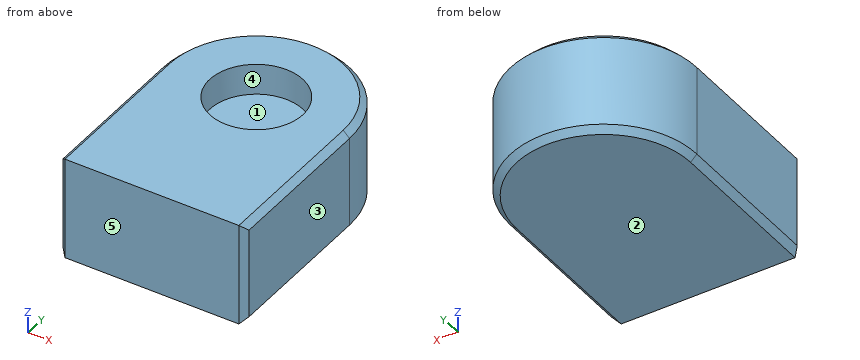
from build123d import *

# Parameters (mm, degrees)
EXTRUDE_1_DEPTH     = 16.5
CHAMFER_1_SIZE      = 1
SKETCH_2_R          = 7.5
CUT_EXTRUDE_1_DEPTH = 5


with BuildPart() as part:
    # 草圖1 → 填料-伸長1 (new body)
    with BuildSketch(Plane.XY):
        with BuildLine():
            Line((-15, 0), (-15, -26))
            Line((-15, -26), (15, -26))
            Line((15, -26), (15, 0))
            ThreePointArc((15, 0), (0, 15), (-15, 0))
        make_face()
    extrude(amount=EXTRUDE_1_DEPTH)

    # 導角1
    chamfer_1_edges = [part.edges().sort_by_distance(p)[0] for p in [
        (15, -13, 16.5),
        (0, 15, 16.5),
        (15, -13, 0),
        (-15, -13, 0),
        (0, 15, 0),
        (-15, -13, 16.5),
        (15, -26, 8.25),
        (-15, -26, 8.25),
    ]]
    chamfer(chamfer_1_edges, length=CHAMFER_1_SIZE)

    # 草圖2 → 除料-伸長1 (cut)
    with BuildSketch(Plane.XY.offset(16.5)):
        Circle(SKETCH_2_R)
    extrude(amount=-CUT_EXTRUDE_1_DEPTH, mode=Mode.SUBTRACT)


solid = part.part
Check sheet for the modelled part. Datum: model origin and axes. Units: mm. Face numbers are marked on the shaded views. A direction names the side the tool comes from. Round coordinates to 2 decimals unless told otherwise and drop trailing zeros. Loops run counter-clockwise (first coordinate to the right, second up) from the corner with the lowest first, then second, coordinate; pieces in that order, holes last.
1. Scan lines: probe 1 along Y at (x, z) = (0, 13.1); probe 2 along Z at (x, y) = (3, 6); probe 3 along X at (y, z) = (0.5, 15.5). Record each from-to range of solid material in increasing order.
2. Sectioned sample at A-A on z = 3. Record the boundary of the cut face in (x, y).
3. Set-up check for the marked faces 1 and 2: record each of +Z, -Z, +X, -X, +Y, -Y from which the full face is reachable in a straight line by a thin tool's end or side.
4. Mould release check, pull along Y, two halves, no side actions. Record for the marked faces 3, 4 and 5: released by +Y, released by -Y, zero draft, split by the parting line, or undercut.
5. Sectioned sample at B-B on x = 0. Record the boundary of the cut face in (y, z).
6. Gauge pin test, flat ends, axial feed: pin 1 Ø3 at (x, z) = (11, 10.5) entering from +Y; pin 2 Ø16.5 at (x, y) = (-2.5, 1) entering from +Z; pin 3 Ø2 at (x, z) = (7, 7) entering from +Y; pin 4 Ø2 at (y, z) = (5, 13) entering from +X. Record the tip position at first contact, or that the pin passes through.
Recorded:
1. probe 1: y = -26 to -7.5, 7.5 to 15
1. probe 2: z = 0 to 11.5
1. probe 3: x = -14.99 to -7.48, 7.48 to 14.99
2. outline: (-15, -25) - (-14, -26) - (14, -26) - (15, -25) - (15, 0) arc R15 ccw to (-15, 0) - close
3. face 1: +Z
3. face 2: -Z, +X, -X, +Y, -Y
4. face 3: zero draft
4. face 4: undercut
4. face 5: released by -Y
5. outline: (-26, 0) - (14, 0) - (15, 1) - (15, 15.5) - (14, 16.5) - (7.5, 16.5) - (7.5, 11.5) - (-7.5, 11.5) - (-7.5, 16.5) - (-26, 16.5) - close
6. pin 1: stops at y = 11.61
6. pin 2: stops at z = 16.5
6. pin 3: stops at y = 13.75
6. pin 4: stops at x = 14.46
